For this review, use the dimensioned drawing (mm, ordinates from the lowest corner) and the shaded views. A direction names the side the tool comes from. Round coordinates to 2 decimals unless told otherwise and drop trailing zeros. Loops run counter-clockwise (first coordinate to the right, second up) from the corner with the lowest first, then second, coordinate; pieces in that order, holes last. Notation, with made-up numbers: M 54,47 L 62,47 A24 ccw 62,85 Z; hole C 28,-36.5 d5. An arc over 180 degrees is marked long. Answer as a JSON object with one key per item and string values. Group by question number.
Item 1: The part is to be moulded in two halves that separate along Y. For the marked faces 3, 4, 5 and 6, say which applies: +Y half, -Y half, draft (parallel to the pull), parting line (faces both ways), or undercut.
Item 2: Tool access review of the marked faces 1 and 2: name each direction out of +Z, -Z, +X, -X, +Y, -Y from which nothing blocks a thin tool from reaching the whole face with its end or side.
Item 3: Consider section D-D (x = 17.5). Give the boundary of the cut face in (y, z).
Item 4: Consider section B-B (x = 13). Give the boundary of the cut face in (y, z).
Item 5: To check wall thickness, follow line 1 (Y direction, x = 14.75, z = 9.75) (1 decimal); line 2 (Y direction, x = 8.5, z = 11.5); line 3 (X direction, y = 5.5, z = 4.75) (1 decimal). State the ranges of each line that lie inside material, in increasing order.
Item 6: Insertion check: P1, Ø2, axis at x = 11.5, z = 5.5, coming from the -Y side; P2, Ø3, axis at x = 3, z = 8.5, coming from the +Y side. Each pin has a flat end and moves straight along its axis. Give the tip position at first contact, or say it passes through.
Item 7: Consider section A-A (z = 1.25). Give the boundary of the cut face in (x, y), and give its area (3 significant figures).
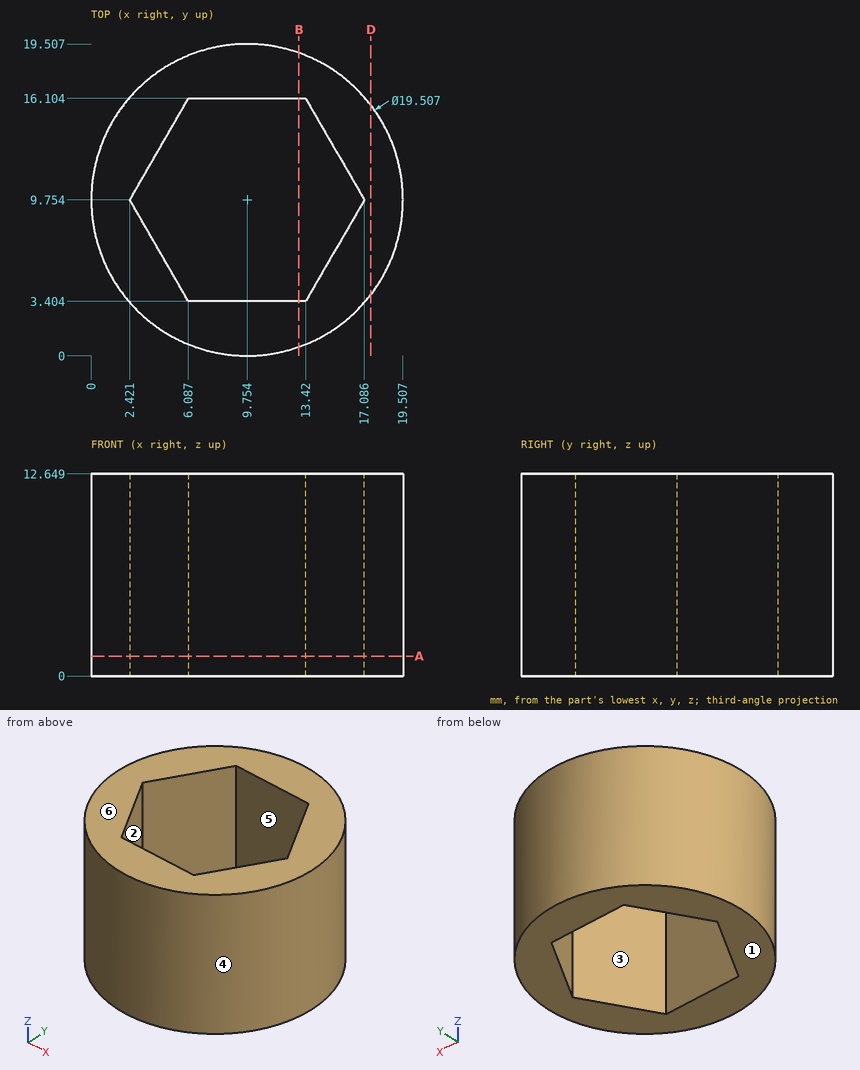
Geometry results:
{
 "1": {"face 3": "undercut", "face 4": "parting line", "face 5": "undercut", "face 6": "draft"},
 "2": {"face 1": "-Z, +X, -X, +Y, -Y", "face 2": "+Z, -Z"},
 "3": {"outline": "M 3.83,0 L 15.68,0 L 15.68,12.65 L 3.83,12.65 Z"},
 "4": {"outline": "M 0.56,0 L 3.4,0 L 3.4,12.65 L 0.56,12.65 Z; M 16.1,0 L 18.95,0 L 18.95,12.65 L 16.1,12.65 Z"},
 "5": {"line 1": "y = 1.4 to 5.7, 13.8 to 18.1", "line 2": "y = 0.08 to 3.4, 16.1 to 19.43", "line 3": "x = 1 to 4.9, 14.6 to 18.5"},
 "6": {"P1": "stops at y = 0.03", "P2": "stops at y = 17.97"},
 "7": {"outline": "C 9.75,9.75 d19.51; hole M 2.42,9.75 L 6.09,3.4 L 13.42,3.4 L 17.09,9.75 L 13.42,16.1 L 6.09,16.1 Z", "area": "159 mm^2"}
}
